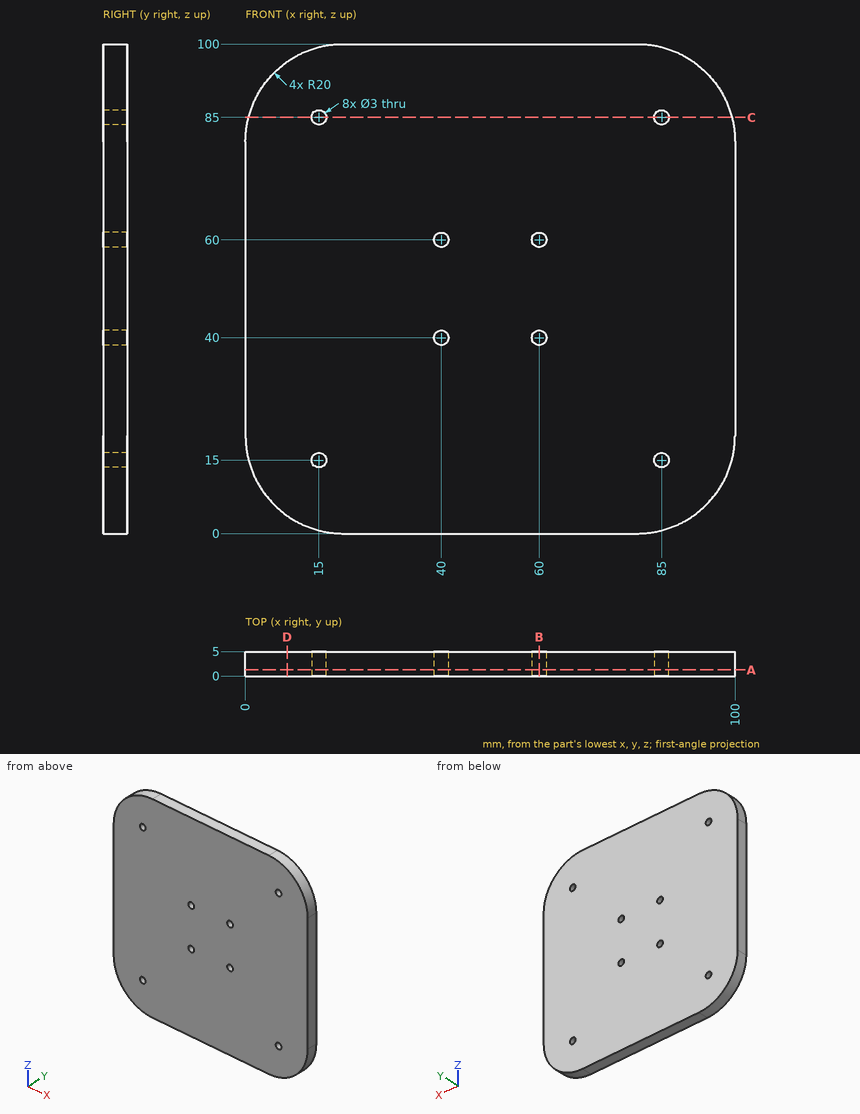
Here's the drawing with two shaded views (mm, measured from the low corner). I have some questions. Coordinates: 2 decimals unless noted, no trailing zeros. Order: outer loops, then holes, each group sorted by start corner. A loop starts at its lowest first (then second) coordinate and runs counter-clockwise, first axis right, second up. Notation, with made-up numbers: (41, -22) - (100, -22) arc R25 cw to (100, 17) - close; hole circle Ø8 at (-28, 6.5). An arc over 180 degrees is marked (long way). Answer in a Markdown table with one row per item. Add a question column.
(1) If we section it at D-D, the plane x = 8.5: Please give me the cut outline in (y, z).
(2) If we section it at C-C, the plane z = 85: Please give me the cut outline in (x, y).
(3) If we section it at A-A, the plane y = 1.25: State how many separate pieces and enclosed holes the cut face has, then the cut area to 3 significant figures.
(4) If we section it at B-B, the plane x = 60: Please give me the cut outline in (y, z), then the cut area to 3 significant figures.
(5) I need wall thicknesses on L1, parallel to X at y = 3.75, z = 60; L2, parallel to X at y = 3.2, z = 15. Which ranges of each line are inside material? Lowest first, please.
(6) Will these pins go through, and if not, where does the flat tip stop? pin 1 (12 mm diameter, centred on x = 55, z = 79, fed in from -Y); pin 2 (2 mm diameter, centred on x = 15.5, y = 3, fed in from +Z); pin 3 (1.8 mm diameter, centred on x = 15, z = 15, fed in from -Y).
Results are:
| question | item | result |
|---|---|---|
| 1 | outline | (0, 3.64) - (5, 3.64) - (5, 96.36) - (0, 96.36) - close |
| 2 | outline | (0.64, 0) - (13.5, 0) - (13.5, 5) - (0.64, 5) - close; (16.5, 0) - (83.5, 0) - (83.5, 5) - (16.5, 5) - close; (86.5, 0) - (99.36, 0) - (99.36, 5) - (86.5, 5) - close |
| 3 | separate pieces | 1 |
| 3 | enclosed holes | 8 |
| 3 | area | 9,600 mm2 |
| 4 | outline | (0, 0) - (5, 0) - (5, 38.5) - (0, 38.5) - close; (0, 41.5) - (5, 41.5) - (5, 58.5) - (0, 58.5) - close; (0, 61.5) - (5, 61.5) - (5, 100) - (0, 100) - close |
| 4 | area | 470 mm2 |
| 5 | L1 | x = 0 to 38.5, 41.5 to 58.5, 61.5 to 100 |
| 5 | L2 | x = 0.64 to 13.5, 16.5 to 83.5, 86.5 to 99.36 |
| 6 | pin 1 | stops at y = 0 |
| 6 | pin 2 | stops at z = 99.69 |
| 6 | pin 3 | passes through |
